```python
from build123d import *

# Parameters (mm, degrees)
F1_DEPTH = 25
F2_R     = 5
F3_T     = -2


with BuildPart() as f1:
    # F0 (on Top) → F1 (new body)
    with BuildSketch(Plane.XY):
        with BuildLine():
            ThreePointArc((26.5, 0), (0, 15.3), (-26.5, 0))
            Line((-26.5, 0), (26.5, 0))
        make_face()
    extrude(amount=F1_DEPTH)

    # F2
    f2_edges = [f1.edges().sort_by_distance(p)[0] for p in [
        (-26.5, 0, 12.5),
        (26.5, 0, 12.5),
    ]]
    fillet(f2_edges, radius=F2_R)

    # F3
    f3_openings = [f1.faces().sort_by_distance(p)[0] for p in [
        (0, 6.722431, 25),
    ]]
    offset(amount=F3_T, openings=f3_openings)


solid = f1.part
```
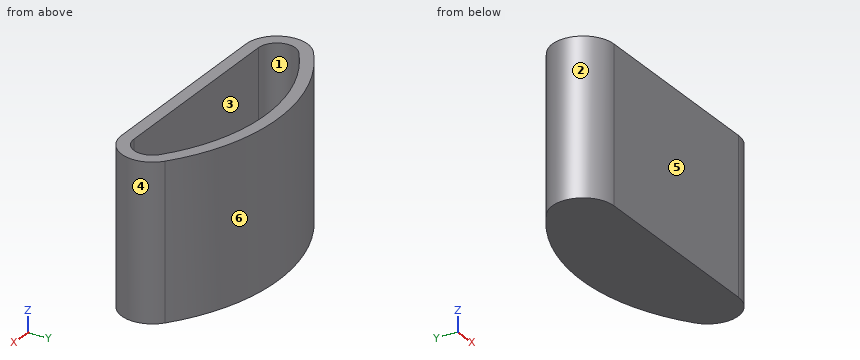
The listing builds one solid part. Answer for the finished solid, in the listing's coordinates (mm). Face numbers are marked on the shaded views. A direction names the side the tool comes from. Give positions to 0.01 mm unless a question says otherwise; leave off trailing zeros. Loops run counter-clockwise (first coordinate to the right, second up) from the corner with the lowest first, then second, coordinate; pieces in that order, holes last. Notation, with made-up numbers: (44, -7.5) - (51, -7.5) arc R28 ccw to (51, 19.5) - close; hole circle Ø4 at (26, 35.5). An arc over 180 degrees is marked (long way). Answer as CSV lines item,"result". Start each with the question number.
Item 1: A cutting plane is placed at C-C on x = -3. Determine the outline of the cut face in (y, z), then the cut area to 3 significant figures.
Item 2: A cutting plane is placed at A-A on y = 5. Determine the outline of the cut face in (x, z).
Item 3: A cutting plane is placed at B-B on z = 22. Determine the outline of the cut face in (x, y).
Item 4: Each of these flat-tipped pins is pushed along its axis until it touches: pin 1 (5 mm diameter, centred on x = 10, z = 15.5, fed in from +Y); pin 2 (8 mm diameter, centred on x = -16.5, z = 5.5, fed in from +Y); pin 3 (6 mm diameter, centred on x = 12, y = 6, fed in from +Z). Where does it stop, or does it pass through?
Item 5: Find the intervals of material crossed by line 1 (X direction, y = 5, z = 16.75); line 2 (Z direction, x = 10.5, y = 8); line 3 (Y direction, x = 17, z = 4.25), in increasing order. Write a range as from..to.
Item 6: The mould has two halves that part along X. Classify the marked faces 3, 4, 5 and 6: +X half, -X half, draft (parallel to the pull), parting line (faces both ways), or undercut.
Item 7: For the marked faces 1 and 2, determine the directions among +Z, -Z, +X, -X, +Y, -Y from which every point of the face is accessible in a straight line to the end or side of a thin tool.
Found:
1,outline,"(0, 0) - (15.15, 0) - (15.15, 25) - (13.14, 25) - (13.14, 2) - (2, 2) - (2, 25) - (0, 25) - close"
1,area,"123 mm^2"
2,outline,"(-20.6, 0) - (20.6, 0) - (20.6, 25) - (18.6, 25) - (18.6, 2) - (-18.6, 2) - (-18.6, 25) - (-20.6, 25) - close"
3,outline,"(-18.64, 8.96) arc R5 ccw to (-15.6, 0) - (15.6, 0) arc R5 ccw to (18.64, 8.96) arc R30.6 ccw to start; hole (-17.42, 7.38) arc R3 ccw to (-15.6, 2) - (15.6, 2) arc R3 ccw to (17.42, 7.38) arc R28.6 ccw to start"
4,pin 1,"stops at y = 14.37"
4,pin 2,"stops at y = 12.63"
4,pin 3,"stops at z = 2"
5,line 1,"x = -20.6..-18.6, 18.6..20.6"
5,line 2,"z = 0..2"
5,line 3,"y = 0.2..2.35, 7.7..10.14"
6,face 3,"undercut"
6,face 4,"+X half"
6,face 5,"draft"
6,face 6,"parting line"
7,face 1,"+Z"
7,face 2,"+Z, -Z, -X"
